```python
from build123d import *

# Parameters (mm, degrees)
SKETCH1_W           = 20
SKETCH1_H           = 35.5
BOSS_EXTRUDE1_DEPTH = 7.25
CUT_EXTRUDE1_DEPTH  = 5.75
SKETCH3_R           = 0.6
CUT_EXTRUDE2_DEPTH  = 7.25
FILLET1_R           = 2
SKETCH4_W           = 2.378205128
SKETCH4_H           = 0.583333334
CUT_EXTRUDE3_DEPTH  = 1
CHAMFER1_SIZE       = 0.5


with BuildPart() as part:
    # Sketch1 → Boss-Extrude1 (new body)
    with BuildSketch(Plane.XY):
        Rectangle(SKETCH1_W, SKETCH1_H)
    extrude(amount=BOSS_EXTRUDE1_DEPTH)

    # Sketch2 → Cut-Extrude1 (cut)
    with BuildSketch(Plane.XY):
        Polygon((-3.625, 11.125), (-3.625, 16.125), (3.625, 16.125), (3.625, 11.125), (8.375, 11.125), (8.375, -11.125), (3.625, -11.125), (3.625, -16.125), (-3.625, -16.125), (-3.625, -11.125), (-8.375, -11.125), (-8.375, 11.125), align=None)
    extrude(amount=CUT_EXTRUDE1_DEPTH, mode=Mode.SUBTRACT)

    # Sketch3 → Cut-Extrude2 (cut)
    with BuildSketch(Plane.XY):
        with Locations((-2.54, -3)):
            Circle(SKETCH3_R)
        with Locations((2.54, -1.984)):
            Circle(SKETCH3_R)
        with Locations((2.54, -4.016)):
            Circle(SKETCH3_R)
    extrude(amount=CUT_EXTRUDE2_DEPTH, mode=Mode.SUBTRACT)

    # Fillet1
    fillet1_edges = [part.edges().sort_by_distance(p)[0] for p in [
        (10, -17.75, 3.625),
        (-10, -17.75, 3.625),
        (-10, 17.75, 3.625),
        (10, 17.75, 3.625),
    ]]
    fillet(fillet1_edges, radius=FILLET1_R)

    # Sketch4 → Cut-Extrude3 (cut)
    with BuildSketch(Plane.XY):
        Polygon((-6.498397436, 14.474358974), (-6.498397436, 15.326923077), (-7.081730769, 15.326923077), (-7.081730769, 14.474358974), (-7.979166667, 14.474358974), (-7.979166667, 13.891025641), (-7.081730769, 13.891025641), (-7.081730769, 13.038461538), (-6.498397436, 13.038461538), (-6.498397436, 13.891025641), (-5.600961538, 13.891025641), (-5.600961538, 14.474358974), align=None)
        with Locations((6.716346154, -14.278846154)):
            Rectangle(SKETCH4_W, SKETCH4_H)
    extrude(amount=CUT_EXTRUDE3_DEPTH, mode=Mode.SUBTRACT)

    # Chamfer1
    chamfer1_edges = [part.edges().sort_by_distance(p)[0] for p in [
        (3.625, 13.625, 0),
        (0, 16.125, 0),
        (-3.625, 13.625, 0),
        (-6, 11.125, 0),
        (-8.375, 0, 0),
        (-6, -11.125, 0),
        (-3.625, -13.625, 0),
        (0, -16.125, 0),
        (3.625, -13.625, 0),
        (6, -11.125, 0),
        (8.375, 0, 0),
        (6, 11.125, 0),
    ]]
    chamfer(chamfer1_edges, length=CHAMFER1_SIZE)


solid = part.part
```
Geometry check sheet. Reference: the model listing, model coordinates, mm. A direction names the side the tool comes from. Coordinates: 2 decimals unless noted, no trailing zeros. Order: outer loops, then holes, each group sorted by start corner. A loop starts at its lowest first (then second) coordinate and runs counter-clockwise, first axis right, second up. Notation, with made-up numbers: (35, 26.25) - (42, 26.25) arc R30 cw to (42, 61.25) - close; hole circle Ø11 at (81, 8). An arc over 180 degrees is marked (long way). Answer in a Markdown table with one row per item. Add a question column.
1. Section check B-B (x = -2.54). Enter the section's corners in (y, z) (3 decimals).
2. Section check A-A (z = 5.25). Enter the section's corners in (x, y) (3 decimals).
3. Section check D-D (x = 2.54). Enter the section's corners in (y, z) (3 decimals).
4. Section check C-C (y = -3). Enter the section's corners in (x, z) (3 decimals).
5. Draft check along Y on faces 1 (the face through (0, 16.125, 3)), 2 (the face through (-9.43, -17.15, 3.68)), 3 (the face through (0, 0, 7.25)). Enter one of: +Y half, -Y half, draft (parallel to the pull), parting line (faces both ways), or undercut.
6. Access from +Z, -Z, +X, -X, +Y, -Y to the whole of each face (thin tool, end or side, straight path). Record for faces 4 (the face through (2.86, -3.51, 6.49)), 5 (the face through (-7.082, 13.5, 0.5)).
7. Material ranges on L1, parallel to Y at x = 2.54, z = 6.75; L2, parallel to X at y = 13, z = 3.25 (3 decimals); L3, parallel to X at y = -3, z = 6.5, recorded low to high. Write a range as [from, to].
8. Gauge pin test, flat end, axial feed: pin 1 Ø10 at (x, y) = (-2.5, 0.5) entering from -Z. Record the tip position at first contact, or that the pin passes through.
Data:
| question | item | result |
|---|---|---|
| 1 | outline | (-17.75, 0) - (-16.625, 0) - (-16.125, 0.5) - (-16.125, 5.75) - (-3.6, 5.75) - (-3.6, 7.25) - (-17.75, 7.25) - close; (-2.4, 5.75) - (16.125, 5.75) - (16.125, 0.5) - (16.625, 0) - (17.75, 0) - (17.75, 7.25) - (-2.4, 7.25) - close |
| 2 | outline | (-10, -15.75) arc R2 ccw to (-8, -17.75) - (8, -17.75) arc R2 ccw to (10, -15.75) - (10, 15.75) arc R2 ccw to (8, 17.75) - (-8, 17.75) arc R2 ccw to (-10, 15.75) - close; hole (-8.375, -11.125) - (-3.625, -11.125) - (-3.625, -16.125) - (3.625, -16.125) - (3.625, -11.125) - (8.375, -11.125) - (8.375, 11.125) - (3.625, 11.125) - (3.625, 16.125) - (-3.625, 16.125) - (-3.625, 11.125) - (-8.375, 11.125) - close |
| 3 | outline | (-17.75, 0) - (-16.625, 0) - (-16.125, 0.5) - (-16.125, 5.75) - (-4.616, 5.75) - (-4.616, 7.25) - (-17.75, 7.25) - close; (-3.416, 5.75) - (-2.584, 5.75) - (-2.584, 7.25) - (-3.416, 7.25) - close; (-1.384, 5.75) - (16.125, 5.75) - (16.125, 0.5) - (16.625, 0) - (17.75, 0) - (17.75, 7.25) - (-1.384, 7.25) - close |
| 4 | outline | (-10, 0) - (-8.875, 0) - (-8.375, 0.5) - (-8.375, 5.75) - (-3.14, 5.75) - (-3.14, 7.25) - (-10, 7.25) - close; (-1.94, 5.75) - (8.375, 5.75) - (8.375, 0.5) - (8.875, 0) - (10, 0) - (10, 7.25) - (-1.94, 7.25) - close |
| 5 | face 1 | undercut |
| 5 | face 2 | -Y half |
| 5 | face 3 | draft |
| 6 | face 4 | +Z, -Z |
| 6 | face 5 | -Z |
| 7 | L1 | y = [-17.75, -4.62], [-3.42, -2.58], [-1.38, 17.75] |
| 7 | L2 | x = [-10, -3.625], [3.625, 10] |
| 7 | L3 | x = [-10, -3.14], [-1.94, 10] |
| 8 | pin 1 | stops at z = 5.75 |
